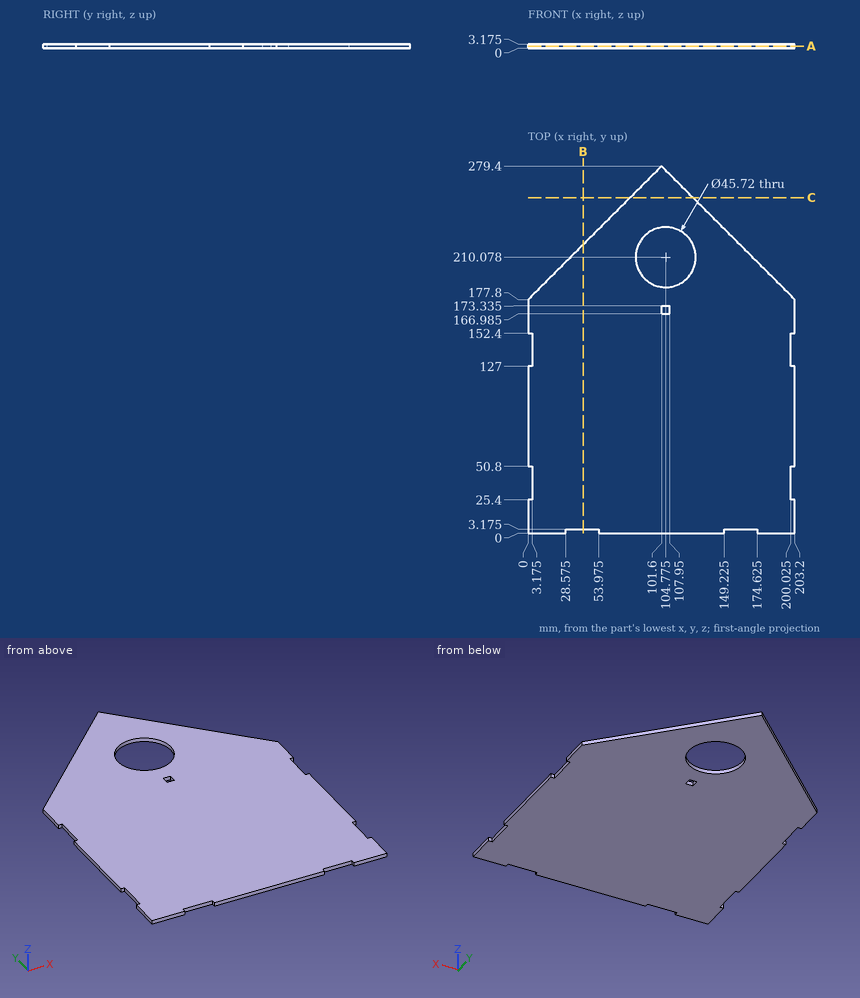
Source: three-view drawing plus pictorial views. Frame: mm from the lowest corner of the part. Coordinates: 2 decimals unless noted, no trailing zeros. Order: outer loops, then holes, each group sorted by start corner. A loop starts at its lowest first (then second) coordinate and runs counter-clockwise, first axis right, second up.
Item 1: Cut plane C-C (y = 255.5). Return loops of the section in (x, z) (1 decimal), plus the area to 3 significant figures.
Output values:
outline: (77.7, 0) - (125.5, 0) - (125.5, 3.2) - (77.7, 3.2) - close
area: 152 mm2
Item 2: Cut plane A-A (z = 1.65). Count the separate pieces of the cut face and the enclosed holes in it, plus the area to 3 significant figures.
Output values:
separate pieces: 1
enclosed holes: 2
area: 44,300 mm2
Item 3: Material intervals for line 1 (Y direction, x = 96, z = 1.9); line 2 (X direction, y = 130.5, z = 0.25) (1 decimal); line 3 (Y direction, x = 89.5, z = 2.3) (1 decimal), sorted ascending.
Output values:
line 1: y = 0 to 188.97, 231.19 to 273.8
line 2: x = 3.2 to 200
line 3: y = 0 to 193.1, 227.1 to 267.3
Item 4: Cut plane B-B (x = 42). Return loops of the section in (y, z) (1 decimal).
Output values:
outline: (3.2, 0) - (219.8, 0) - (219.8, 3.2) - (3.2, 3.2) - close
Item 5: First-contact query: P1, Ø1.5, axis at x = 32.5, z = 1.5, coming from the +Y side; P2, Ø1.6, axis at y = 144.5, z = 1, coming from the +X side (3 decimals); P3, Ø1.6, axis at x = 167.5, z = 2, coming from the -Y side (3 decimals). Flat tips, straight axial feed; report the tip coordinate or a pass-through.
Output values:
P1: stops at y = 211.05
P2: stops at x = 200.025
P3: stops at y = 3.175
